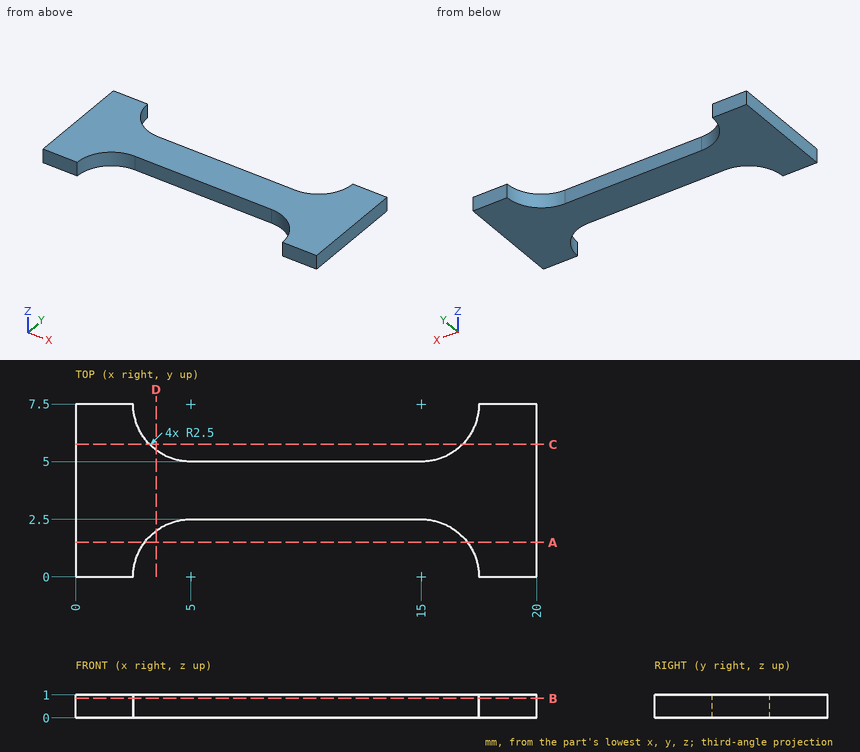
Geometry check sheet. Reference: drawing and pictorial views, mm from the part's lowest x, y, z. Coordinates: 2 decimals unless noted, no trailing zeros. Order: outer loops, then holes, each group sorted by start corner. A loop starts at its lowest first (then second) coordinate and runs counter-clockwise, first axis right, second up. Notation, with made-up numbers: (44.25, -39.5) - (56.25, -39.5) arc R21 cw to (56.25, -24.5) - close; hole circle Ø10 at (9, 79). An arc over 180 degrees is marked (long way). Answer in a Markdown table with one row per item. Add a question column.
1) Material ranges on line 1 along Y through (x, z) = (11.5, 0.15); line 2 along X through (y, z) = (5.25, 0.5); line 3 along X through (y, z) = (6, 0.55), recorded low to high. Write a range as [from, to].
2) Cross-section at A-A, the plane y = 1.5. Record the cut outline in (x, z), then the cut area to 3 significant figures.
3) Cross-section at B-B, the plane z = 0.85. Record the cut outline in (x, y), then the cut area to 3 significant figures.
4) Cross-section at D-D, the plane x = 3.5. Record the cut outline in (y, z).
5) Cross-section at C-C, the plane y = 5.75. Record the cut outline in (x, z), then the cut area to 3 significant figures.
Check result:
| question | item | result |
|---|---|---|
| 1 | line 1 | y = [2.5, 5] |
| 1 | line 2 | x = [0, 3.91], [16.09, 20] |
| 1 | line 3 | x = [0, 3], [17, 20] |
| 2 | outline | (0, 0) - (3, 0) - (3, 1) - (0, 1) - close; (17, 0) - (20, 0) - (20, 1) - (17, 1) - close |
| 2 | area | 6.00 mm² |
| 3 | outline | (0, 0) - (2.5, 0) arc R2.5 cw to (5, 2.5) - (15, 2.5) arc R2.5 cw to (17.5, 0) - (20, 0) - (20, 7.5) - (17.5, 7.5) arc R2.5 cw to (15, 5) - (5, 5) arc R2.5 cw to (2.5, 7.5) - (0, 7.5) - close |
| 3 | area | 80.4 mm² |
| 4 | outline | (2, 0) - (5.5, 0) - (5.5, 1) - (2, 1) - close |
| 5 | outline | (0, 0) - (3.21, 0) - (3.21, 1) - (0, 1) - close; (16.79, 0) - (20, 0) - (20, 1) - (16.79, 1) - close |
| 5 | area | 6.43 mm² |
